The listing builds one solid part. Answer for the finished solid, in the listing's coordinates (mm). Face numbers are marked on the shaded views. Round coordinates to 2 decimals unless told otherwise and drop trailing zeros. Loops run counter-clockwise (first coordinate to the right, second up) from the corner with the lowest first, then second, coordinate; pieces in that order, holes last. Notation, with made-up numbers: M 10.5,6 L 14.5,6 A9 cw 14.5,20 Z; hole C 49.25,-8 d9. An arc over 180 degrees is marked long. Put each result on its own line as item: value. Start each with the question number.
(1) A flat-ended cylindrical pin translates along its axis: P1, Ø2, axis at x = -25.5, y = 22, coming from the +Z side. Find the tip coordinate at first contact, or state that the pin passes through.
(2) Section B-B, the plane y = 0 is taken. Determine the outline of the cut face in (x, z), then the cut area to 3 significant figures.
(3) Section A-A, the plane z = -6 is taken. Determine the outline of the cut face in (x, y), then the cut area to 3 significant figures.
(4) Straight lines are drawn through the part: line 1 (Y direction, x = 0, z = -4); line 2 (Z direction, x = -6, y = -17.5); line 3 (X direction, y = -19.5, z = -5.25). For each, find the intervals that lie inside material, in ascending order.
(5) Determine the mould class of the marked faces 1, 2 and 3 for opening direction Y: released by +Y, released by -Y, zero draft, split by the parting line, or undercut.
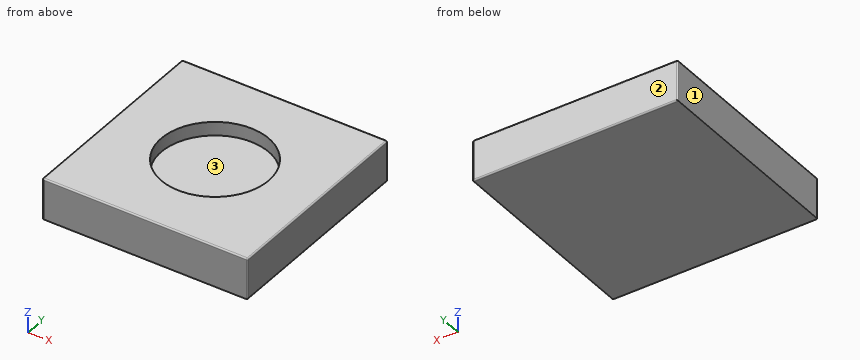
```python
from build123d import *

# Parameters (mm, degrees)
SKETCH1_W           = 150
SKETCH1_H           = 150
BOSS_EXTRUDE1_DEPTH = 30
FILLET1_R           = 1
SKETCH2_R           = 39.25
CUT_EXTRUDE4_DEPTH  = 10


with BuildPart() as part:
    # Sketch1 → Boss-Extrude1 (new body)
    with BuildSketch(Plane.XY):
        Rectangle(SKETCH1_W, SKETCH1_H)
    extrude(amount=-BOSS_EXTRUDE1_DEPTH)

    # Fillet1
    fillet1_edges = [part.edges().sort_by_distance(p)[0] for p in [
        (0, 75, -30),
        (-75, 0, 0),
        (0, 75, 0),
        (75, 0, 0),
        (0, -75, 0),
        (-75, -75, -15),
        (-75, 75, -15),
        (75, 75, -15),
        (75, -75, -15),
        (75, 0, -30),
    ]]
    fillet(fillet1_edges, radius=FILLET1_R)

    # Sketch2 → Cut-Extrude4 (cut)
    with BuildSketch(Plane.XY):
        Circle(SKETCH2_R)
    extrude(amount=-CUT_EXTRUDE4_DEPTH, mode=Mode.SUBTRACT)


solid = part.part
```
Recorded:
1. P1: stops at z = -10
2. outline: M -75,-30 L 74,-30 A1 ccw 75,-29 L 75,-1 A1 ccw 74,0 L 39.25,0 L 39.25,-10 L -39.25,-10 L -39.25,0 L -74,0 A1 ccw -75,-1 Z
2. area: 3,710 mm²
3. outline: M -75,-74 A1 ccw -74,-75 L 74,-75 A1 ccw 75,-74 L 75,74 A1 ccw 74,75 L -74,75 A1 ccw -75,74 Z; hole C 0,0 d78.5
3. area: 17,700 mm²
4. line 1: y = -75 to -39.25, 39.25 to 75
4. line 2: z = -30 to -10
4. line 3: x = -75 to -34.06, 34.06 to 75
5. face 1: zero draft
5. face 2: released by +Y
5. face 3: undercut
